from build123d import *

# Parameters (mm, degrees)
SKETCH1_R           = 32
BOSS_EXTRUDE1_DEPTH = 13
SKETCH2_R           = 27
CUT_EXTRUDE1_DEPTH  = 7
SKETCH3_R           = 2.5
CUT_EXTRUDE2_DEPTH  = 46.793012567
SKETCH4_R           = 3.5
CUT_EXTRUDE3_DEPTH  = 5
BOSS_EXTRUDE2_START = 7
SKETCH7_R           = 27
SKETCH7_R_2         = 26
BOSS_EXTRUDE2_DEPTH = 7
SKETCH8_R           = 11
CUT_EXTRUDE6_DEPTH  = 46.793012567
FILLET2_R           = 0.5
SKETCH10_R          = 32
BOSS_EXTRUDE3_DEPTH = 13
SKETCH11_R          = 2
CUT_EXTRUDE9_DEPTH  = 52.176166328
FILLET3_R           = 0.5
SKETCH5_R           = 2
CUT_EXTRUDE11_DEPTH = 52.176166464
CUT_EXTRUDE12_DEPTH = 3


with BuildPart() as part:
    # Sketch1 → Boss-Extrude1 (new body)
    with BuildSketch(Plane(origin=(0, 0, 0), x_dir=(1, 0, 0), z_dir=(0, 1, 0))):
        with Locations(Location((0, 0, 0), (0, 0, 90))):
            Circle(SKETCH1_R)
    extrude(amount=BOSS_EXTRUDE1_DEPTH)

    # Sketch2 → Cut-Extrude1 (cut)
    with BuildSketch(Plane(origin=(0, 13, 0), x_dir=(1, 0, 0), z_dir=(0, 1, 0))):
        with Locations(Location((0, 0, 0), (0, 0, 270))):
            Circle(SKETCH2_R)
    extrude(amount=-CUT_EXTRUDE1_DEPTH, mode=Mode.SUBTRACT)

    # Sketch3 → Cut-Extrude2 (cut, through all)
    with BuildSketch(Plane(origin=(0, 6, 0), x_dir=(1, 0, 0), z_dir=(0, 1, 0))):
        with Locations(Location((-14.849242405, 14.849242405, 0), (0, 0, 270))):
            Circle(SKETCH3_R)
        with Locations(Location((14.849242405, 14.849242405, 0), (0, 0, 270))):
            Circle(SKETCH3_R)
        with Locations(Location((14.849242405, -14.849242405, 0), (0, 0, 270))):
            Circle(SKETCH3_R)
        with Locations(Location((-14.849242405, -14.849242405, 0), (0, 0, 270))):
            Circle(SKETCH3_R)
    extrude(amount=-CUT_EXTRUDE2_DEPTH, mode=Mode.SUBTRACT)

    # Sketch4 → Cut-Extrude3 (cut)
    with BuildSketch(Plane(origin=(0, 6, 0), x_dir=(1, 0, 0), z_dir=(0, 1, 0))):
        with Locations(Location((-14.849242405, 14.849242405, 0), (0, 0, 270))):
            Circle(SKETCH4_R)
        with Locations(Location((14.849242405, 14.849242405, 0), (0, 0, 270))):
            Circle(SKETCH4_R)
        with Locations(Location((14.849242405, -14.849242405, 0), (0, 0, 270))):
            Circle(SKETCH4_R)
        with Locations(Location((-14.849242405, -14.849242405, 0), (0, 0, 270))):
            Circle(SKETCH4_R)
    extrude(amount=-CUT_EXTRUDE3_DEPTH, mode=Mode.SUBTRACT)

    # Sketch7 → Boss-Extrude2 (add)
    with BuildSketch(Plane(origin=(0, 6, 0), x_dir=(1, 0, 0), z_dir=(0, 1, 0)).offset(BOSS_EXTRUDE2_START)):
        Circle(SKETCH7_R)
        with Locations(Location((0, 0, 0), (0, 0, 270))):
            Circle(SKETCH7_R_2, mode=Mode.SUBTRACT)
    extrude(amount=-BOSS_EXTRUDE2_DEPTH)

    # Sketch8 → Cut-Extrude6 (cut, through all)
    with BuildSketch(Plane(origin=(0, 6, 0), x_dir=(1, 0, 0), z_dir=(0, 1, 0))):
        with Locations(Location((0, 0, 0), (0, 0, 270))):
            Circle(SKETCH8_R)
    extrude(amount=-CUT_EXTRUDE6_DEPTH, mode=Mode.SUBTRACT)

    # Fillet2
    fillet2_edges = [part.edges().sort_by_distance(p)[0] for p in [
        (0, 0, -11),
        (0, 6, -11),
    ]]
    fillet(fillet2_edges, radius=FILLET2_R)

    # Sketch10 → Boss-Extrude3 (add)
    with BuildSketch(Plane(origin=(0, 0, 0), x_dir=(1, 0, 0), z_dir=(0, 1, 0))):
        with BuildLine():
            Line((10.355339059, 35), (-10.355339059, 35))
            ThreePointArc((-10.355339059, 35), (-14.182173383, 34.238795325), (-17.426406871, 32.071067812))
            Line((-17.426406871, 32.071067812), (-32.071067812, 17.426406871))
            ThreePointArc((-32.071067812, 17.426406871), (-34.238795325, 14.182173383), (-35, 10.355339059))
            Line((-35, 10.355339059), (-35, -10.355339059))
            ThreePointArc((-35, -10.355339059), (-34.238795325, -14.182173383), (-32.071067812, -17.426406871))
            Line((-32.071067812, -17.426406871), (-17.426406871, -32.071067812))
            ThreePointArc((-17.426406871, -32.071067812), (-14.182173383, -34.238795325), (-10.355339059, -35))
            Line((-10.355339059, -35), (10.355339059, -35))
            ThreePointArc((10.355339059, -35), (14.182173383, -34.238795325), (17.426406871, -32.071067812))
            Line((17.426406871, -32.071067812), (32.071067812, -17.426406871))
            ThreePointArc((32.071067812, -17.426406871), (34.238795325, -14.182173383), (35, -10.355339059))
            Line((35, -10.355339059), (35, 10.355339059))
            ThreePointArc((35, 10.355339059), (34.238795325, 14.182173383), (32.071067812, 17.426406871))
            Line((32.071067812, 17.426406871), (17.426406871, 32.071067812))
            ThreePointArc((17.426406871, 32.071067812), (14.182173383, 34.238795325), (10.355339059, 35))
        make_face()
        Circle(SKETCH10_R, mode=Mode.SUBTRACT)
    extrude(amount=BOSS_EXTRUDE3_DEPTH)

    # Sketch11 → Cut-Extrude9 (cut, through all)
    with BuildSketch(Plane(origin=(0, 13, 0), x_dir=(1, 0, 0), z_dir=(0, 1, 0))):
        with Locations(Location((-21.566756826, 21.566756826, 0), (0, 0, 270))):
            Circle(SKETCH11_R)
        with Locations(Location((21.566756826, 21.566756826, 0), (0, 0, 270))):
            Circle(SKETCH11_R)
        with Locations(Location((21.566756826, -21.566756826, 0), (0, 0, 270))):
            Circle(SKETCH11_R)
        with Locations(Location((-21.566756826, -21.566756826, 0), (0, 0, 270))):
            Circle(SKETCH11_R)
    extrude(amount=-CUT_EXTRUDE9_DEPTH, mode=Mode.SUBTRACT)

    # Fillet3
    fillet3_edges = [part.edges().sort_by_distance(p)[0] for p in [
        (-14.182173383, 0, 34.238795325),
        (0, 0, 35),
        (14.182173383, 0, 34.238795325),
        (24.748737342, 0, 24.748737342),
        (34.238795325, 0, 14.182173383),
        (35, 0, 0),
        (34.238795325, 0, -14.182173383),
        (24.748737342, 0, -24.748737342),
        (14.182173383, 0, -34.238795325),
        (0, 0, -35),
        (-14.182173383, 0, -34.238795325),
        (-24.748737342, 0, -24.748737342),
        (-34.238795325, 0, -14.182173383),
        (-35, 0, 0),
        (-34.238795325, 0, 14.182173383),
        (-24.748737342, 0, 24.748737342),
    ]]
    fillet(fillet3_edges, radius=FILLET3_R)

    # Sketch5 → Cut-Extrude11 (cut, through all)
    with BuildSketch(Plane(origin=(0, 13, 0), x_dir=(1, 0, 0), z_dir=(0, 1, 0))):
        with Locations(Location((0, 30.5, 0), (0, 0, 270))):
            Circle(SKETCH5_R)
        with Locations(Location((30.5, 0, 0), (0, 0, 270))):
            Circle(SKETCH5_R)
        with Locations(Location((0, -30.5, 0), (0, 0, 270))):
            Circle(SKETCH5_R)
        with Locations(Location((-30.5, 0, 0), (0, 0, 270))):
            Circle(SKETCH5_R)
    extrude(amount=-CUT_EXTRUDE11_DEPTH, mode=Mode.SUBTRACT)

    # Sketch12 → Cut-Extrude12 (cut)
    with BuildSketch(Plane.XZ):
        Polygon((-3.175426481, 30.5), (-1.58771324, 27.75), (1.58771324, 27.75), (3.175426481, 30.5), (1.58771324, 33.25), (-1.58771324, 33.25), align=None)
        Polygon((-30.5, -3.175426481), (-27.75, -1.58771324), (-27.75, 1.58771324), (-30.5, 3.175426481), (-33.25, 1.58771324), (-33.25, -1.58771324), align=None)
        Polygon((30.5, 3.175426481), (27.75, 1.58771324), (27.75, -1.58771324), (30.5, -3.175426481), (33.25, -1.58771324), (33.25, 1.58771324), align=None)
        Polygon((3.175426481, -30.5), (1.58771324, -27.75), (-1.58771324, -27.75), (-3.175426481, -30.5), (-1.58771324, -33.25), (1.58771324, -33.25), align=None)
    extrude(amount=-CUT_EXTRUDE12_DEPTH, mode=Mode.SUBTRACT)


solid = part.part
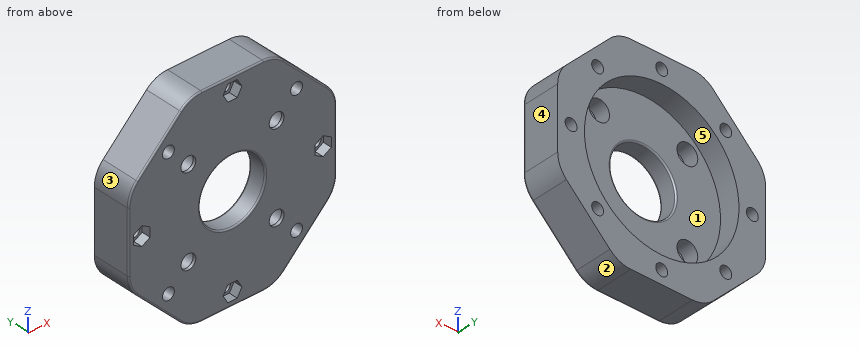
Work out the finished part from the listing and answer in its coordinate system (mm). Face numbers are marked on the shaded views. A direction names the side the tool comes from. Give positions to 0.01 mm unless a question says otherwise; leave off trailing zeros. Use a Markdown table: item, result. Add a question column.
1. For the marked faces 1 and 2, determine the directions among +Z, -Z, +X, -X, +Y, -Y from which every point of the face is accessible in a straight line to the end or side of a thin tool.
2. Find the intervals of material crossed by probe 1 along X at (y, z) = (2.45, 0); probe 2 along Z at (x, y) = (1, 5.75); probe 3 along Y at (x, z) = (-21.5, 11), in increasing order.
3. Section A-A on x = 0 is taken. State how many separate pieces and enclosed holes the cut face has, and give its area (3 significant figures).
4. Determine the mould class of the marked faces 3, 4 and 5 for opening direction Z: released by +Z, released by -Z, zero draft, split by the parting line, or undercut.
5. Flat-ended cylindrical pins translate along their axes: pin 1 Ø17.5 at (x, z) = (0, 0) entering from -Y; pin 2 Ø6.5 at (x, z) = (-21.57, -21.57) entering from +Y; pin 3 Ø1.5 at (y, z) = (1.5, -14.5) entering from +X; pin 4 Ø4 at (x, y) = (-13, 2.5) entering from +Z. Find the tip coordinate at first contact, or state that the pin passes through.
Results below:
| question | item | result |
|---|---|---|
| 1 | face 1 | +Y |
| 1 | face 2 | -Z, +X, +Y, -Y |
| 2 | probe 1 | x = -35 to -33.25, -27.75 to -11, 11 to 27.75, 33.25 to 35 |
| 2 | probe 2 | z = -35 to -32.23, -28.77 to -11.02, 11.02 to 28.77, 32.23 to 35 |
| 2 | probe 3 | y = 0 to 6 |
| 3 | separate pieces | 4 |
| 3 | enclosed holes | 0 |
| 3 | area | 301 mm^2 |
| 4 | face 3 | released by +Z |
| 4 | face 4 | zero draft |
| 4 | face 5 | undercut |
| 5 | pin 1 | passes through |
| 5 | pin 2 | stops at y = 13 |
| 5 | pin 3 | stops at x = 34.41 |
| 5 | pin 4 | stops at z = 34.98 |
